Work out the finished part from the listing and answer in its coordinate system (mm). Coordinates: 2 decimals unless noted, no trailing zeros. Write each loop counter-clockwise with the first axis right and the second up, starting at its lowest first coordinate (ties: lowest second). Pieces come first, ordered by that corner, then holes. Notation, with made-up numbers: (-32.75, 12.25) - (26.25, 12.25) arc R36 ccw to (26.25, 46.25) - close; hole circle Ø6 at (-10.75, 3). An arc over 180 degrees is marked (long way). Use a Markdown table: item, result. Add a question column.
(1) The part is cut by section B-B, the plane y = 0.95. State how many separate pieces and enclosed holes the cut face has, then the cut area to 3 significant figures.
(2) Find the intervals of material crossed by line 1 (X direction, y = 1.2, z = -103); line 2 (X direction, y = 0.35, z = -78.5); line 3 (Z direction, x = 132.1, y = 0.8), in increasing order. Write a range as from..to.
(3) Given pin 1 Ø5 at (x, z) = (107, -17) entering from -Y; pin 2 Ø1.9 at (x, z) = (132.1, -6) entering from +Y, each flat-ended and moving along its own axis, determine where each tip first touches the part or whether it passes through.
(4) The part is cut by section A-A, the plane z = -68.5. Give the vertices of the cut face in (x, y).
from build123d import *

# Parameters (mm, degrees)
SKETCH1_W           = 138.1
SKETCH1_H           = 109
SKETCH1_R           = 1.6
SKETCH1_W_2         = 30
SKETCH1_H_2         = 3.2
SKETCH1_W_3         = 3.2
SKETCH1_H_3         = 24
SKETCH1_W_4         = 19.101
SKETCH1_H_4         = 8.153
BOSS_EXTRUDE1_DEPTH = 2
FILLET1_R           = 6
FILLET2_R           = 6
FILLET3_R           = 6


with BuildPart() as part:
    # Sketch1 → Boss-Extrude1 (new body)
    with BuildSketch(Plane(origin=(0, 0, 0), x_dir=(1, 0, 0), z_dir=(0, 1, 0))):
        with Locations((69.05, 54.5)):
            Rectangle(SKETCH1_W, SKETCH1_H)
        with Locations(Location((6, 103, 0), (0, 0, 270))):
            Circle(SKETCH1_R, mode=Mode.SUBTRACT)
        with Locations(Location((132.1, 103, 0), (0, 0, 270))):
            Circle(SKETCH1_R, mode=Mode.SUBTRACT)
        with Locations(Location((132.1, 6, 0), (0, 0, 270))):
            Circle(SKETCH1_R, mode=Mode.SUBTRACT)
        with Locations(Location((6, 6, 0), (0, 0, 270))):
            Circle(SKETCH1_R, mode=Mode.SUBTRACT)
        with Locations((47, 5.414130674)):
            Rectangle(SKETCH1_W_2, SKETCH1_H_2, mode=Mode.SUBTRACT)
        with Locations((47, 103)):
            Rectangle(SKETCH1_W_2, SKETCH1_H_2, mode=Mode.SUBTRACT)
        with Locations((91.1, 103)):
            Rectangle(SKETCH1_W_2, SKETCH1_H_2, mode=Mode.SUBTRACT)
        with Locations((91.1, 5.414130674)):
            Rectangle(SKETCH1_W_2, SKETCH1_H_2, mode=Mode.SUBTRACT)
        with Locations((6, 76)):
            Rectangle(SKETCH1_W_3, SKETCH1_H_3, mode=Mode.SUBTRACT)
        with Locations((6, 33)):
            Rectangle(SKETCH1_W_3, SKETCH1_H_3, mode=Mode.SUBTRACT)
        with Locations((132.1, 76)):
            Rectangle(SKETCH1_W_3, SKETCH1_H_3, mode=Mode.SUBTRACT)
        with Locations((132.1, 33)):
            Rectangle(SKETCH1_W_3, SKETCH1_H_3, mode=Mode.SUBTRACT)
        with Locations((100.3195, 86.8275)):
            Rectangle(SKETCH1_W_4, SKETCH1_H_4, mode=Mode.SUBTRACT)
    extrude(amount=BOSS_EXTRUDE1_DEPTH)

    # Fillet1
    fillet1_edges = [part.edges().sort_by_distance(p)[0] for p in [
        (0, 1, -109),
    ]]
    fillet(fillet1_edges, radius=FILLET1_R)

    # Fillet2
    fillet2_edges = [part.edges().sort_by_distance(p)[0] for p in [
        (0, 1, 0),
    ]]
    fillet(fillet2_edges, radius=FILLET2_R)

    # Fillet3
    fillet3_edges = [part.edges().sort_by_distance(p)[0] for p in [
        (138.1, 1, -109),
        (138.1, 1, 0),
    ]]
    fillet(fillet3_edges, radius=FILLET3_R)


solid = part.part
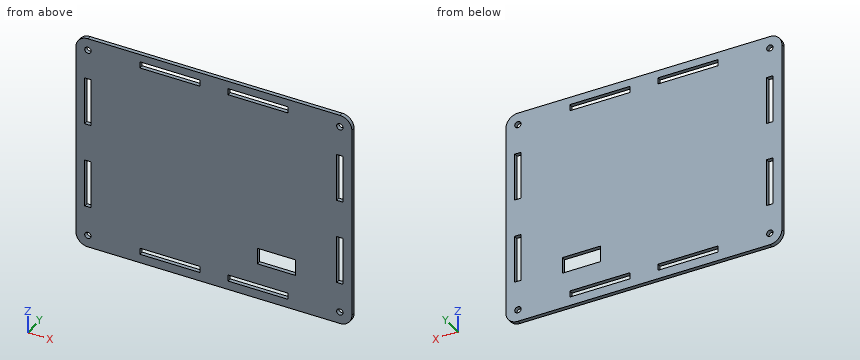
Model answer:
| question | item | result |
|---|---|---|
| 1 | separate pieces | 1 |
| 1 | enclosed holes | 13 |
| 1 | area | 14,100 mm^2 |
| 2 | line 1 | 0..4.4, 7.6..32, 62..76.1, 106.1..130.5, 133.7..138.1 |
| 2 | line 2 | 0..4.4, 7.6..130.5, 133.7..138.1 |
| 2 | line 3 | -109..-104.6, -101.4..-88, -64..-45, -21..-7.6, -4.4..0 |
| 3 | pin 1 | y = 0 |
| 3 | pin 2 | through |
| 4 | outline | (0, 0) - (4.4, 0) - (4.4, 2) - (0, 2) - close; (7.6, 0) - (130.5, 0) - (130.5, 2) - (7.6, 2) - close; (133.7, 0) - (138.1, 0) - (138.1, 2) - (133.7, 2) - close |
